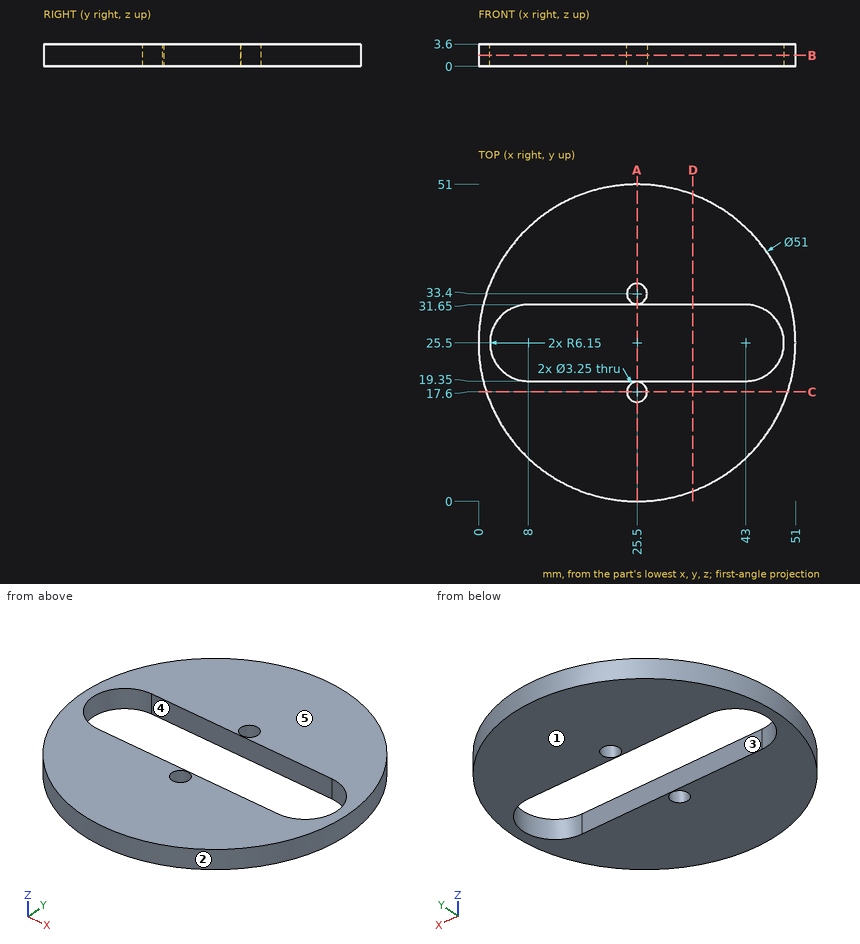
Input: dimensioned drawing with shaded views. Units: mm. Origin: part minimum x, y, z. A direction names the side the tool comes from. Round coordinates to 2 decimals unless told otherwise and drop trailing zeros. Order: outer loops, then holes, each group sorted by start corner. A loop starts at its lowest first (then second) coordinate and runs counter-clockwise, first axis right, second up.
1. Cut plane B-B, the plane z = 1.75. Output: boundary loops of the cut face in (x, y) (3 decimals).
The answers:
outline: circle Ø51 at (25.5, 25.5); hole (8, 19.35) - (43, 19.35) arc R6.15 ccw to (43, 31.65) - (8, 31.65) arc R6.15 ccw to start; hole circle Ø3.25 at (25.5, 17.6); hole circle Ø3.25 at (25.5, 33.4)
2. Cut plane D-D, the plane x = 34.5. Output: boundary loops of the cut face in (y, z).
The answers:
outline: (1.64, 0) - (19.35, 0) - (19.35, 3.6) - (1.64, 3.6) - close; (31.65, 0) - (49.36, 0) - (49.36, 3.6) - (31.65, 3.6) - close
3. Cut plane A-A, the plane x = 25.5. Output: boundary loops of the cut face in (y, z) (3 decimals).
The answers:
outline: (0, 0) - (15.975, 0) - (15.975, 3.6) - (0, 3.6) - close; (19.225, 0) - (19.35, 0) - (19.35, 3.6) - (19.225, 3.6) - close; (31.65, 0) - (31.775, 0) - (31.775, 3.6) - (31.65, 3.6) - close; (35.025, 0) - (51, 0) - (51, 3.6) - (35.025, 3.6) - close
4. Material intervals for line 1 (Y direction, x = 25, z = 0.3); line 2 (Y direction, x = 43, z = 3.1); line 3 (Y direction, x = 41, z = 1.9), sorted ascending.
The answers:
line 1: y = 0 to 16.05, 19.15 to 19.35, 31.65 to 31.85, 34.95 to 51
line 2: y = 6.95 to 19.35, 31.65 to 44.05
line 3: y = 5.25 to 19.35, 31.65 to 45.75
5. Cut plane C-C, the plane y = 17.6. Output: boundary loops of the cut face in (x, z) (3 decimals), then the cut area to 3 significant figures.
The answers:
outline: (1.255, 0) - (23.875, 0) - (23.875, 3.6) - (1.255, 3.6) - close; (27.125, 0) - (49.745, 0) - (49.745, 3.6) - (27.125, 3.6) - close
area: 163 mm2
6. Set-up query: the marked faces 4 and 5. Return all of +Z, -Z, +X, -X, +Y, -Y with unobstructed straight access to the full face (end or side cutting, diameter ignored); none if empty.
The answers:
face 4: +Z, -Z
face 5: +Z, +X, -X, +Y, -Y
7. Mould query, pull axis Y, two halves, no side actions, for the marked faces 1, 2 and 3. Classes: released by +Y, released by -Y, zero draft, split by the parting line, or undercut.
The answers:
face 1: zero draft
face 2: split by the parting line
face 3: undercut
8. Pin query (flat end, axial travel): P1, Ø1, axis at y = 30.5, z = 1.5, coming from the -X side; P2, Ø1.8, axis at x = 28, z = 2, coming from the +Y side; P3, Ø1, axis at y = 9.5, z = 0.5, coming from the -X side. Return the tip coordinate at first contact, or that it passes through.
The answers:
P1: stops at x = 0.4
P2: stops at y = 50.95
P3: stops at x = 5.25
